Geometry check sheet. Reference: the model listing, model coordinates, mm. Round coordinates to 2 decimals unless told otherwise and drop trailing zeros. Write each loop counter-clockwise with the first axis right and the second up, starting at its lowest first coordinate (ties: lowest second). Pieces come first, ordered by that corner, then holes.
Item 1: Cross-section at A-A (z = 0). Enter the section's corners in (x, y), then the cut area to 3 significant figures.
Item 2: Scan lines: probe 1 along Z at (x, y) = (-0.5, 1); probe 2 along X at (y, z) = (3.5, 54.5) (3 decimals); probe 3 along Z at (x, y) = (4.5, 2.5). Record each from-to range of solid material in increasing order.
Item 3: Depth check by flat-ended pin: P1, Ø21.5, axis at x = -107.823, z = 0, coming from the -Y side; P2, Ø1, axis at y = 5.5, z = -22.5, coming from the -X side; P3, Ø1, axis at y = 5, z = 64.5, coming from the +X side; P4, Ø8, axis at x = 0, z = -107.823, coming from the -Y side. Enter the tip coordinate at first touch or a pass-through.
Item 4: Cross-section at B-B (x = 0). Enter the section's corners in (y, z).
Item 5: Cross-section at C-C (y = 1.5). State how many separate pieces and enclosed holes the cut face has, then the cut area to 3 significant figures.
Item 6: Draft check along X on faces 1 (the face through (3.11, 3.13, -113.81)), 2 (the face through (-190.4, 3.1, 2)), 3 (the face through (190.57, 3.13, -1.37)). Enter one of: pulls with the +X half, pulls with the -X half, needs draft (parallel to the pull), parting line crosses it, or undercut.
from build123d import *

# Parameters (mm, degrees)
F0_R     = 6.74624
F1_DEPTH = 6.35
F2_R     = 90.17
F3_DEPTH = 6.351
F4_R     = 6.74624
F5_DEPTH = 6.351
F6_R     = 0.508


with BuildPart() as f1:
    # F0 (on Front) → F1 (new body)
    with BuildSketch(Plane.XZ):
        with BuildLine():
            ThreePointArc((-196.5166448066, -120.3328961324), (-194.775442891, -125.0265791688), (-190.1745674547, -127))
            Line((-190.1745674547, -127), (190.1745674547, -127))
            ThreePointArc((190.1745674547, -127), (194.775442891, -125.0265791688), (196.5166448066, -120.3328961324))
            Line((196.5166448066, -120.3328961324), (184.4516448066, 120.9671038676))
            ThreePointArc((184.4516448066, 120.9671038676), (182.4861466235, 125.2508754362), (178.1095674547, 127))
            Line((178.1095674547, 127), (-178.1095674547, 127))
            ThreePointArc((-178.1095674547, 127), (-182.4861466235, 125.2508754362), (-184.4516448066, 120.9671038676))
            Line((-184.4516448066, 120.9671038676), (-196.5166448066, -120.3328961324))
        make_face()
        with Locations((-173.0375, -85.725)):
            Circle(F0_R, mode=Mode.SUBTRACT)
        with Locations((173.0375, -85.725)):
            Circle(F0_R, mode=Mode.SUBTRACT)
        with Locations((-166.6875, 60.325)):
            Circle(F0_R, mode=Mode.SUBTRACT)
        with Locations((166.6875, 60.325)):
            Circle(F0_R, mode=Mode.SUBTRACT)
    extrude(amount=-F1_DEPTH)

    # F2 (on face) → F3 (cut, through all)
    with BuildSketch(Plane.XZ):
        Circle(F2_R)
    extrude(amount=-F3_DEPTH, mode=Mode.SUBTRACT)

    # F4 (on face) → F5 (cut, through all)
    with BuildSketch(Plane.XZ):
        with Locations((0, 107.823)):
            Circle(F4_R)
        with Locations((-107.823, 0)):
            Circle(F4_R)
        with Locations((0, -107.823)):
            Circle(F4_R)
        with Locations((107.823, 0)):
            Circle(F4_R)
    extrude(amount=-F5_DEPTH, mode=Mode.SUBTRACT)

    # F6
    f6_edges = [f1.edges().sort_by_distance(p)[0] for p in [
        (-90.17, 6.35, 0),
        (-90.17, 0, 0),
    ]]
    fillet(f6_edges, radius=F6_R)


solid = f1.part
Resolved:
1. outline: (-190.5, 0) - (-114.57, 0) - (-114.57, 6.35) - (-190.5, 6.35) - close; (-101.08, 0) - (-90.68, 0) arc R0.51 ccw to (-90.17, 0.51) - (-90.17, 5.84) arc R0.51 ccw to (-90.68, 6.35) - (-101.08, 6.35) - close; (90.17, 0.51) arc R0.51 ccw to (90.68, 0) - (101.08, 0) - (101.08, 6.35) - (90.68, 6.35) arc R0.51 ccw to (90.17, 5.84) - close; (114.57, 0) - (190.5, 0) - (190.5, 6.35) - (114.57, 6.35) - close
1. area: 1,100 mm2
2. probe 1: z = -127 to -114.55, -101.1 to -90.17, 90.17 to 101.1, 114.55 to 127
2. probe 2: x = -187.775 to -170.091, -163.284 to -71.836, 71.836 to 163.284, 170.091 to 187.775
2. probe 3: z = -127 to -112.85, -102.8 to -90.06, 90.06 to 102.8, 112.85 to 127
3. P1: stops at y = 0
3. P2: stops at x = -191.65
3. P3: stops at x = 187.3
3. P4: passes through
4. outline: (0, -127) - (6.35, -127) - (6.35, -114.57) - (0, -114.57) - close; (0, -101.08) - (6.35, -101.08) - (6.35, -90.68) arc R0.51 ccw to (5.84, -90.17) - (0.51, -90.17) arc R0.51 ccw to (0, -90.68) - close; (0, 90.68) arc R0.51 ccw to (0.51, 90.17) - (5.84, 90.17) arc R0.51 ccw to (6.35, 90.68) - (6.35, 101.08) - (0, 101.08) - close; (0, 114.57) - (6.35, 114.57) - (6.35, 127) - (0, 127) - close
5. separate pieces: 1
5. enclosed holes: 9
5. area: 70,100 mm2
6. face 1: undercut
6. face 2: pulls with the -X half
6. face 3: pulls with the +X half
